from build123d import *

# Parameters (mm, degrees)
CROQUIS1_W              = 15
CROQUIS1_H              = 10
CROQUIS1_R              = 1
SALIENTE_EXTRUIR1_DEPTH = 10
CROQUIS2_R              = 1
CORTAR_EXTRUIR1_DEPTH   = 10
REDONDEO1_R             = 1


with BuildPart() as part:
    # Croquis1 → Saliente-Extruir1 (new body)
    with BuildSketch(Plane.XY):
        with Locations((-10.722064782, 5.272312164)):
            Rectangle(CROQUIS1_W, CROQUIS1_H)
        with Locations((-10.722064782, 5.272312164)):
            Circle(CROQUIS1_R, mode=Mode.SUBTRACT)
    extrude(amount=SALIENTE_EXTRUIR1_DEPTH)

    # Croquis2 → Cortar-Extruir1 (cut)
    with BuildSketch(Plane(origin=(0, 10.272312164, 0), x_dir=(-1, 0, 0), z_dir=(0, 1, 0))):
        with Locations(Location((15.722064782, 5, 0), (0, 0, 90))):
            Circle(CROQUIS2_R)
        with Locations(Location((5.722064782, 5, 0), (0, 0, 90))):
            Circle(CROQUIS2_R)
    extrude(amount=-CORTAR_EXTRUIR1_DEPTH, mode=Mode.SUBTRACT)

    # Redondeo1
    redondeo1_edges = [part.edges().sort_by_distance(p)[0] for p in [
        (-3.222064782, 5.272312164, 10),
        (-18.222064782, 5.272312164, 10),
        (-3.222064782, 5.272312164, 0),
        (-18.222064782, 5.272312164, 0),
    ]]
    fillet(redondeo1_edges, radius=REDONDEO1_R)


solid = part.part
Read the model definition and answer for the solid it produces. Units are mm, in the model's axes. Give positions to 0.01 mm unless a question says otherwise; leave off trailing zeros. Write each loop counter-clockwise with the first axis right and the second up, starting at its lowest first coordinate (ties: lowest second). Pieces come first, ordered by that corner, then holes. Notation, with made-up numbers: (-11, -13.75) - (26, -13.75) arc R23 cw to (26, -3.75) - close; hole circle Ø5 at (-26.75, 35). An arc over 180 degrees is marked (long way). Use CSV: the item, a comma, the result in double quotes. Start each with the question number.
Item 1: Consider line 1 (X direction, y = 8.75, z = 5); line 2 (Z direction, x = -6.25, y = 1.25); line 3 (Z direction, x = -15, y = 1.5). Determine where each line is inside the solid, lowest interval first.
Item 2: The part is cut by section C-C, the plane x = -15.5. Give the vertices of the cut face in (y, z), and give its area (3 significant figures).
Item 3: The part is cut by section D-D, the plane y = 7. Give the vertices of the cut face in (x, z), and give its area (3 significant figures).
Item 4: The part is cut by section B-B, the plane z = 5.25. Give the vertices of the cut face in (x, y).
Item 5: The mould has two halves that part along X. Classify faces 1 (the cylindrical face through (-16.61, 5.34, 5.46)), 2 (the flat face through (-11, 10.272, 5)), 3 (the cylindrical face through (-17.937, 5.342, 9.699)), 4 (the cylindrical face through (-6.7, 5.3, 4.8)): pulls with the +X half, pulls with the -X half, needs draft (parallel to the pull), parting line crosses it, or undercut.
Item 6: The part is cut by section A-A, the plane y = 5.5. Give the vertices of the cut face in (x, z), and give its area (3 significant figures).
Taken from the geometry:
1,line 1,"-18.22 to -16.72, -14.72 to -6.72, -4.72 to -3.22"
1,line 2,"0 to 4.15, 5.85 to 10"
1,line 3,"0 to 4.31, 5.69 to 10"
2,outline,"(0.27, 0) - (10.27, 0) - (10.27, 4.02) - (0.27, 4.02) - close; (0.27, 5.98) - (10.27, 5.98) - (10.27, 10) - (0.27, 10) - close"
2,area,"80.5 mm2"
3,outline,"(-18.22, 1) arc R1 ccw to (-17.22, 0) - (-4.22, 0) arc R1 ccw to (-3.22, 1) - (-3.22, 9) arc R1 ccw to (-4.22, 10) - (-17.22, 10) arc R1 ccw to (-18.22, 9) - close; hole circle Ø2 at (-15.72, 5); hole circle Ø2 at (-5.72, 5)"
3,area,"143 mm2"
4,outline,"(-18.22, 0.27) - (-16.69, 0.27) - (-16.69, 10.27) - (-18.22, 10.27) - close; (-14.75, 0.27) - (-6.69, 0.27) - (-6.69, 10.27) - (-14.75, 10.27) - close; (-4.75, 0.27) - (-3.22, 0.27) - (-3.22, 10.27) - (-4.75, 10.27) - close; hole circle Ø2 at (-10.72, 5.27)"
5,face 1,"undercut"
5,face 2,"needs draft"
5,face 3,"pulls with the -X half"
5,face 4,"undercut"
6,outline,"(-18.22, 1) arc R1 ccw to (-17.22, 0) - (-11.7, 0) - (-11.7, 10) - (-17.22, 10) arc R1 ccw to (-18.22, 9) - close; (-9.75, 0) - (-4.22, 0) arc R1 ccw to (-3.22, 1) - (-3.22, 9) arc R1 ccw to (-4.22, 10) - (-9.75, 10) - close; hole circle Ø2 at (-15.72, 5); hole circle Ø2 at (-5.72, 5)"
6,area,"123 mm2"
